Read the model definition and answer for the solid it produces. Units are mm, in the model's axes. A direction names the side the tool comes from. Round coordinates to 2 decimals unless told otherwise and drop trailing zeros. Write each loop counter-clockwise with the first axis right and the second up, starting at its lowest first coordinate (ties: lowest second). Pieces come first, ordered by that corner, then holes. Notation, with made-up numbers: M 30.25,-8 L 45.25,-8 A16 cw 45.25,13 Z; hole C 43,61 d1. An arc over 180 degrees is marked long. Use one line per item in the form item = value. Start each with the question number.
```python
from build123d import *

# Parameters (mm, degrees)
SKETCH1_R           = 2.54
BOSS_EXTRUDE1_DEPTH = 5.715
SKETCH2_R           = 1.1303
BOSS_EXTRUDE2_DEPTH = 12.065
SKETCH4_R           = 3.175
BOSS_EXTRUDE3_DEPTH = 2.54
SKETCH3_W           = 2.54
SKETCH3_H           = 2.54
CUT_EXTRUDE1_DEPTH  = 2.286
FILLET1_R           = 0.254


with BuildPart() as part:
    # Sketch1 → Boss-Extrude1 (new body)
    with BuildSketch(Plane(origin=(0, 0, 0), x_dir=(1, 0, 0), z_dir=(0, 1, 0))):
        with Locations(Location((0, 0, 0), (0, 0, 270))):
            Circle(SKETCH1_R)
    extrude(amount=-BOSS_EXTRUDE1_DEPTH)

    # Sketch2 → Boss-Extrude2 (add)
    with BuildSketch(Plane(origin=(0, 0, 0), x_dir=(1, 0, 0), z_dir=(0, 1, 0))):
        with Locations(Location((0, 0, 0), (0, 0, 270))):
            Circle(SKETCH2_R)
    extrude(amount=-BOSS_EXTRUDE2_DEPTH)

    # Sketch4 → Boss-Extrude3 (add)
    with BuildSketch(Plane(origin=(0, 0, 0), x_dir=(1, 0, 0), z_dir=(0, 1, 0))):
        with Locations(Location((0, 0, 0), (0, 0, 270))):
            Circle(SKETCH4_R)
    extrude(amount=-BOSS_EXTRUDE3_DEPTH)

    # Sketch3 → Cut-Extrude1 (cut)
    with BuildSketch(Plane(origin=(0, 0, 0), x_dir=(1, 0, 0), z_dir=(0, 1, 0))):
        Rectangle(SKETCH3_W, SKETCH3_H)
    extrude(amount=-CUT_EXTRUDE1_DEPTH, mode=Mode.SUBTRACT)

    # Fillet1
    fillet1_edges = [part.edges().sort_by_distance(p)[0] for p in [
        (0, -2.54, -3.175),
        (0, 0, -3.175),
    ]]
    fillet(fillet1_edges, radius=FILLET1_R)


solid = part.part
```
Q1. For a pull along Z with two mould halves and no side action, classify faces 4 (the face through (0, -12.065, 0)), 5 (the face through (0.34, -8.85, 1.08)), 6 (the face through (0, -1, 1.27)) as +Z half, -Z half, draft (parallel to the pull), parting line (faces both ways), or undercut.
Q2. Find section A-A on z = 0. Write down the section's boundary in (x, y) (3 decimals).
Q3. A tool of negligible diameter and unlimited length cuts with its end or side. For faces 1 (the face through (-1.93, -1.26, -2.52)), 2 (the face through (2.52, -4.11, -0.33)), 3 (the face through (0, -2.286, 0)), from which of +Z, -Z, +X, -X, +Y, -Y can it reach the whole face along a straight path? Write none if from no direction.
Q4. Find section B-B on x = 0. Write down the section's boundary in (y, z) (3 decimals), and give its area (3 significant figures).
Q5. Straight lines are drawn through the part: line 1 (Y direction, x = -0.75, z = 2.5); line 2 (X direction, y = -9.75, z = 0); line 3 (Y direction, x = 0.25, z = -0.25) (3 decimals). For each, find the intervals that lie inside material, in ascending order. Write a range as [from, to].
Q6. Each of these flat-tipped pins is pushed along its axis until it touches: pin 1 Ø1.3 at (x, z) = (0, 0) entering from +Y; pin 2 Ø3 at (x, y) = (1.5, -9.5) entering from +Z; pin 3 Ø1.1 at (x, y) = (0.5, -1.5) entering from +Z (3 decimals). Where does it stop, or does it pass through?
Q7. Find section D-D on y = -5. Write down the section's boundary in (x, z).
Q8. Find section C-C on y = -2. Write down the section's boundary in (x, z) (3 decimals), and give its area (3 significant figures).
Response:
q1.face_4 = draft
q1.face_5 = parting line
q1.face_6 = undercut
q2.outline = M -3.175,-2.286 A0.254 ccw -2.921,-2.54 L -2.54,-2.54 L -2.54,-5.715 L -1.13,-5.715 L -1.13,-12.065 L 1.13,-12.065 L 1.13,-5.715 L 2.54,-5.715 L 2.54,-2.54 L 2.921,-2.54 A0.254 ccw 3.175,-2.286 L 3.175,-0.254 A0.254 ccw 2.921,0 L 1.27,0 L 1.27,-2.286 L -1.27,-2.286 L -1.27,0 L -2.921,0 A0.254 ccw -3.175,-0.254 Z
q3.face_1 = +Y, -Y
q3.face_2 = -Y
q3.face_3 = +Y
q4.outline = M -12.065,-1.13 L -5.715,-1.13 L -5.715,-2.54 L -2.54,-2.54 L -2.54,-2.921 A0.254 ccw -2.286,-3.175 L -0.254,-3.175 A0.254 ccw 0,-2.921 L 0,-1.27 L -2.286,-1.27 L -2.286,1.27 L 0,1.27 L 0,2.921 A0.254 ccw -0.254,3.175 L -2.286,3.175 A0.254 ccw -2.54,2.921 L -2.54,2.54 L -5.715,2.54 L -5.715,1.13 L -12.065,1.13 Z
q4.area = 40.8 mm²
q5.line_1 = [-2.54, 0]
q5.line_2 = [-1.13, 1.13]
q5.line_3 = [-12.065, -2.286]
q6.pin_1 = -2.29
q6.pin_2 = 1.13
q6.pin_3 = 3.175
q7.outline = C 0,0 d5.08
q8.outline = C 0,0 d6.35; hole M -1.27,-1.27 L 1.27,-1.27 L 1.27,1.27 L -1.27,1.27 Z
q8.area = 25.2 mm²
